```python
from build123d import *

# Parameters (mm, degrees)
F0_R     = 7.25
F1_DEPTH = 88
F2_R     = 4
F3_DEPTH = 22
F4_SIZE  = 1
F5_R     = 1.75
F6_DEPTH = 120
F7_R     = 5
F8_DEPTH = 78


with BuildPart() as f1:
    # F0 (on Front) → F1 (new body)
    with BuildSketch(Plane.XZ):
        Circle(F0_R)
    extrude(amount=F1_DEPTH)

    # F2 (on Front) → F3 (join)
    with BuildSketch(Plane.XZ):
        Circle(F2_R)
    extrude(amount=-F3_DEPTH)

    # F4
    f4_edges = [f1.edges().sort_by_distance(p)[0] for p in [
        (-4, 22, 0),
    ]]
    chamfer(f4_edges, length=F4_SIZE)

    # F5 (on face) → F6 (cut)
    with BuildSketch(Plane(origin=(0, 22, 0), x_dir=(-1, 0, 0), z_dir=(0, 1, 0))):
        Circle(F5_R)
    extrude(amount=-F6_DEPTH, mode=Mode.SUBTRACT)

    # F7 (on face) → F8 (cut)
    with BuildSketch(Plane.XZ.offset(88)):
        Circle(F7_R)
    extrude(amount=-F8_DEPTH, mode=Mode.SUBTRACT)


solid = f1.part
```
The model under review builds one solid part; all positions refer to its coordinate system, in mm. A direction names the side the tool comes from. Round coordinates to 2 decimals unless told otherwise and drop trailing zeros. Loops run counter-clockwise (first coordinate to the right, second up) from the corner with the lowest first, then second, coordinate; pieces in that order, holes last. Notation, with made-up numbers: M 34,-25.5 L 60,-25.5 A16 ccw 60,-17.5 Z; hole C -2,30 d5. An arc over 180 degrees is marked long. Put each result on its own line as item: value.
Q1. Consider section D-D, the plane y = -5. Give the boundary of the cut face in (x, z), then the cut area to 3 significant figures.
Result set:
outline: C 0,0 d14.5; hole C 0,0 d3.5
area: 156 mm²
Q2. Mouldability with a two-part tool opening along Z and no side actions: class faces 1 (the cylindrical face through (3.35, -43.38, -6.43)), 2 (the cylindrical face through (-1.08, -49.55, -4.88)), 3 (the flat face through (0, 22, -2)) as released by +Z, released by -Z, zero draft, split by the parting line, or undercut.
Result set:
face 1: split by the parting line
face 2: undercut
face 3: zero draft
Q3. Machinability: for faces 4 (the flat face through (0, -10, -2)), 5 (the cylindrical face through (-0.867, 10.353, -3.905)), 6 (the flat face through (-2, -88, -5)), which of the approach directions +Z, -Z, +X, -X, +Y, -Y give a long, thin tool a straight path to every point of the face, cutting with its end or side? Answer none if there is none.
Result set:
face 4: -Y
face 5: +Y
face 6: +Z, -Z, +X, -X, -Y
Q4. For pin 1 (1 mm diameter, centred on y = 5.5, z = 1, fed in from -X); pin 2 (1 mm diameter, centred on x = 2.5, y = -37.5, fed in from -Z); pin 3 (1.5 mm diameter, centred on x = 2, y = -48, fed in from -Z); pin 4 (3 mm diameter, centred on x = 0, z = 0, fed in from -Y), all flat-tipped, find the tip position at first contact; note any pin that passes through.
Result set:
pin 1: stops at x = -3.97
pin 2: stops at z = -6.97
pin 3: stops at z = -7.14
pin 4: passes through
Q5. Consider section B-B, the plane x = 0. Give the boundary of the cut face in (y, z), then the cut area to 3 significant figures.
Result set:
outline: M -88,-7.25 L 0,-7.25 L 0,-4 L 21,-4 L 22,-3 L 22,-1.75 L -10,-1.75 L -10,-5 L -88,-5 Z; M -88,5 L -10,5 L -10,1.75 L 22,1.75 L 22,3 L 21,4 L 0,4 L 0,7.25 L -88,7.25 Z
area: 559 mm²
Q6. To check wall thickness, follow L1, parallel to Z at x = 0, y = -29.5; L2, parallel to Y at x = -1, z = -1.5; L3, parallel to Z at x = -5.25, y = -13.5. State the ranges of each line that lie inside material, in increasing order.
Result set:
L1: z = -7.25 to -5, 5 to 7.25
L2: y = -10 to 22
L3: z = -5 to 5
Q7. Consider section C-C, the plane y = -77. Give the boundary of the cut face in (x, z).
Result set:
outline: C 0,0 d14.5; hole C 0,0 d10
Q8. Consider section A-A, the plane z = 0. Give the boundary of the cut face in (x, y).
Result set:
outline: M -7.25,-88 L -5,-88 L -5,-10 L -1.75,-10 L -1.75,22 L -3,22 L -4,21 L -4,0 L -7.25,0 Z; M 1.75,-10 L 5,-10 L 5,-88 L 7.25,-88 L 7.25,0 L 4,0 L 4,21 L 3,22 L 1.75,22 Z
